from build123d import *

# Parameters (mm, degrees)
SKETCH1_R           = 3
BOSS_EXTRUDE1_DEPTH = 1
FILLET1_R           = 3
BOSS_EXTRUDE2_DEPTH = 1


with BuildPart() as part:
    # Sketch1 → Boss-Extrude1 (new body)
    with BuildSketch(Plane.XY):
        Polygon((-4.515055907, -5.207968635), (4.515055907, -5.207968635), (4.515055907, 6.442798737), (7.135711465, 6.442798737), (0, 13.578510202), (-7.135711465, 6.442798737), (-4.515055907, 6.442798737), align=None)
        Circle(SKETCH1_R, mode=Mode.SUBTRACT)
    extrude(amount=BOSS_EXTRUDE1_DEPTH)

    # Fillet1
    fillet1_edges = [part.edges().sort_by_distance(p)[0] for p in [
        (4.515055907, -5.207968635, 0.5),
        (-4.515055907, -5.207968635, 0.5),
    ]]
    fillet(fillet1_edges, radius=FILLET1_R)

    # Sketch2 → Boss-Extrude2 (add)
    with BuildSketch(Plane(origin=(0, 0, 0), x_dir=(-1, 0, 0), z_dir=(0, 0, -1))):
        with BuildLine():
            ThreePointArc((0, 3), (0.507305936, 2.956795679), (1, 2.828427125))
            Line((1, 2.828427125), (1, 4.210117693))
            Line((1, 4.210117693), (0, 4.210117693))
            Line((0, 4.210117693), (0, 3))
        make_face()
        with BuildLine():
            ThreePointArc((-1, 2.828427125), (-0.507305936, 2.956795679), (0, 3))
            Line((0, 3), (0, 4.210117693))
            Line((0, 4.210117693), (-1, 4.210117693))
            Line((-1, 4.210117693), (-1, 2.828427125))
        make_face()
    extrude(amount=BOSS_EXTRUDE2_DEPTH)


solid = part.part
Part model, mm, in its own coordinate system. A direction names the side the tool comes from. Coordinates: 2 decimals unless noted, no trailing zeros. Loops run counter-clockwise (first coordinate to the right, second up) from the corner with the lowest first, then second, coordinate; pieces in that order, holes last. Notation, with made-up numbers: M -17,37 L 29,37 A21 cw 29,59 Z; hole C -15,60 d8. An arc over 180 degrees is marked long. Use a Markdown table: item, result. Add a question column.
Q1. Pin check, flat tips, straight feed: P1, Ø3, axis at x = -1, y = 1.5, coming from the -Z side; P2, Ø0.5, axis at y = 3, z = 0.5, coming from the +X side; P3, Ø0.5, axis at y = 3, z = 0.5, coming from the -X side; P4, Ø0.8, axis at y = 3.5, z = -0.5, coming from the -X side. Stop position of each tip, or through.
Q2. Cut at A-A (y = 0). Write the cut outline in (x, z), and give its area (3 significant figures).
Q3. Which spindle directions (+Z, -Z, +X, -X, +Y, -Y) get a long thin tool onto all of the face, cutting with end or side? Do faces 1 (the flat face through (4.515, 2.1, 0.5)), 2 (the flat face through (-1, 3.5, -0.5)), 3 (the flat face through (0, 4.21, -0.5)), 4 (the flat face through (-4.515, 2.2, 0.5)), 5 (the flat face through (1, 3.5, -0.5)). Say none if no direction does.
Q4. Probe L1, parallel to X at y = 0, z = 0.4; L2, parallel to Z at x = -4.5, y = 8.5; L3, parallel to X at y = 3.75, z = 0.5. List the from-to ranges inside material, lowest first.
Q5. Cut at C-C (x = 0.5). Write the cut outline in (y, z), and give its area (3 significant figures).
Q6. Cut at D-D (z = -0.25). Write the cut outline in (x, y), and give its area (3 significant figures).
Q7. Cut at B-B (z = 0.65). Write the cut outline in (x, y).
Worked out:
| question | item | result |
|---|---|---|
| 1 | P1 | stops at z = -1 |
| 1 | P2 | stops at x = 4.52 |
| 1 | P3 | stops at x = -4.52 |
| 1 | P4 | stops at x = -1 |
| 2 | outline | M -4.52,0 L -3,0 L -3,1 L -4.52,1 Z; M 3,0 L 4.52,0 L 4.52,1 L 3,1 Z |
| 2 | area | 3.03 mm2 |
| 3 | face 1 | +Z, -Z, +X, -Y |
| 3 | face 2 | -Z, -X, +Y, -Y |
| 3 | face 3 | -Z, +X, -X, +Y |
| 3 | face 4 | +Z, -Z, -X, -Y |
| 3 | face 5 | -Z, +X, +Y, -Y |
| 4 | L1 | x = -4.52 to -3, 3 to 4.52 |
| 4 | L2 | z = 0 to 1 |
| 4 | L3 | x = -4.52 to 4.52 |
| 5 | outline | M -5.21,0 L -2.96,0 L -2.96,1 L -5.21,1 Z; M 2.96,-1 L 4.21,-1 L 4.21,0 L 13.08,0 L 13.08,1 L 2.96,1 Z |
| 5 | area | 13.6 mm2 |
| 6 | outline | M -1,2.83 A3 cw 1,2.83 L 1,4.21 L -1,4.21 Z |
| 6 | area | 2.53 mm2 |
| 7 | outline | M -7.14,6.44 L -4.52,6.44 L -4.52,-2.21 A3 ccw -1.52,-5.21 L 1.52,-5.21 A3 ccw 4.52,-2.21 L 4.52,6.44 L 7.14,6.44 L 0,13.58 Z; hole C 0,0 d6 |
